Autodesk Inventor part; units mm, degrees
ref_plane "YZ Plane" through (0, 0, 0) normal (1, 0, 0) x (0, 1, 0)
ref_plane "XZ Plane" through (0, 0, 0) normal (0, 1, 0) x (-1, 0, 0)
ref_plane "XY Plane" through (0, 0, 0) normal (0, 0, 1) x (1, 0, 0)
sketch "Esquisse1" plane through (0, 0, 0) normal (0, 1, 0) x (-1, 0, 0)
  line L0 (0, 0) -> (-40, 0)
  line L1 (-40, 0) -> (-40, -80)
  line L2 (-40, -80) -> (0, -80)
  line L3 (0, -80) -> (0, 0)
  dimension "d0" = 80
  dimension "d4" = 40
extrude "Extrusion1" add sketch "Esquisse1" along normal blind 80
sketch "Esquisse2" plane through (40, 0, 0) normal (1, 0, 0) x (0, 0, -1)
  point P0 (0, 0)
sketch "Esquisse3" plane through (40, 0, 0) normal (1, 0, 0) x (0, 0, -1)
  line L0 (0, 80) -> (80, 80)
  line L1 (20, 20) -> (60, 20)
  line L2 (60, 20) -> (60, 80)
  line L3 (60, 80) -> (20, 80)
  line L4 (20, 80) -> (20, 20)
  line L5 (0, 0) -> (80, 0)
  line L6 (80, 0) -> (80, 80)
  line L7 (0, 0) -> (0, 80)
  point P0 (20, 80)
  dimension "d9" = 20
  dimension "d10" = 20
  dimension "d11" = 20
extrude "Extrusion2" cut sketch "Esquisse3" against normal blind 80 contours L0 L2 L1 L4
sketch "Esquisse4" plane through (40, 20, -20) normal (0, 1, 0) x (1, 0, 0)
  line L0 (0, 40) -> (-40, 40)
  line L1 (0, 0) -> (-5, 0)
  line L2 (-5, 40) -> (0, 40)
  line L3 (0, 40) -> (0, 0)
  line L4 (-5, 40) -> (-10, 40)
  line L5 (-9, 10) -> (-12, 10)
  line L6 (-12, 10) -> (-12, 30)
  line L7 (-12, 30) -> (-9, 30)
  line L8 (-9, 10) -> (-9, 30)
  point P0 (-40, -20)
  dimension "d19" = 20
  dimension "d21" = 9
  dimension "d22" = 3
extrude "Extrusion3" cut sketch "Esquisse4" against normal blind 10
sketch "Esquisse6" plane through (40, 20, -20) normal (0, 0, -1) x (-1, 0, 0)
  line L0 (40, 60) -> (40, 0)
  line L1 (0, 60) -> (40, 60)
  line L2 (0, 0) -> (0, 60)
  line L3 (0, 0) -> (40, 0)
  point P0 (40, -20)
extrude "Extrusion4" add sketch "Esquisse6" along normal blind 9
sketch "Esquisse7" plane through (40, 20, -60) normal (0, 0, 1) x (1, 0, 0)
  line L0 (-40, 0) -> (-40, 60)
  line L1 (0, 0) -> (-40, 0)
  line L2 (0, 60) -> (0, 0)
  line L3 (-40, 60) -> (0, 60)
  point P0 (-40, -20)
extrude "Extrusion5" add sketch "Esquisse7" along normal blind 9
properties part number "Intsragam"
Work out the finished part from the listing and answer in its coordinate system (mm). A direction names the side the tool comes from. Coordinates: 2 decimals unless noted, no trailing zeros. Write each loop counter-clockwise with the first axis right and the second up, starting at its lowest first coordinate (ties: lowest second). Pieces come first, ordered by that corner, then holes. Notation, with made-up numbers: M 53.5,22.25 L 106.5,22.25 A17 cw 106.5,37.25 Z; hole C 81.25,75.5 d5. An arc over 180 degrees is marked long. Use one line per item in the form item = value. Start each with the question number.
1. The mould has two halves that part along X. Classify faces 4 (the face through (40, 41, -58)), 5 (the face through (20, 39, 0)), 6 (the face through (28, 15, -40)): released by +X, released by -X, zero draft, split by the parting line, or undercut.
2. Straight lines are drawn through the part: probe 1 along Z at (x, y) = (17.5, 45.5); probe 2 along Y at (x, z) = (23.5, -40.5). For each, find the intervals that lie inside material, in ascending order. Write a range as from..to.
3. The part is cut by section D-D (x = 29.5). Give the vertices of the cut face in (y, z).
4. The part is cut by section B-B (z = -40). Give the vertices of the cut face in (x, y).
5. A tool of negligible diameter and unlimited length cuts with its end or side. For faces 1 (the face through (20, 80, -66)), 2 (the face through (29, 10, -40)), 3 (the face through (20, 50, -29)), from which of +Z, -Z, +X, -X, +Y, -Y can it reach the whole face along a straight path? Write none if from no direction.
6. This flat-tipped pin is pushed along its axis until it touches: P1, Ø11, axis at x = 20, z = -40, coming from the +Y side. Where does it stop, or does it pass through?
7. The part is cut by section A-A (y = 17). Give the vertices of the cut face in (x, z).
8. The part is cut by section C-C (y = 68). Give the vertices of the cut face in (x, z), plus the area to 3 significant figures.
Evaluation:
q1.face_4 = released by +X
q1.face_5 = zero draft
q1.face_6 = undercut
q2.probe_1 = -80..-51, -29..0
q2.probe_2 = 0..20
q3.outline = M 0,-80 L 80,-80 L 80,-51 L 20,-51 L 20,-50 L 10,-50 L 10,-30 L 20,-30 L 20,-29 L 80,-29 L 80,0 L 0,0 Z
q4.outline = M 0,0 L 40,0 L 40,20 L 31,20 L 31,10 L 28,10 L 28,20 L 0,20 Z
q5.face_1 = +Z, -Z, +X, -X, +Y
q5.face_2 = +Y
q5.face_3 = +X, -X, +Y
q6.P1 = 20
q7.outline = M 0,-80 L 40,-80 L 40,0 L 0,0 Z; hole M 28,-50 L 31,-50 L 31,-30 L 28,-30 Z
q8.outline = M 0,-80 L 40,-80 L 40,-51 L 0,-51 Z; M 0,-29 L 40,-29 L 40,0 L 0,0 Z
q8.area = 2,320 mm^2
